Geometry: final body of the model. Coordinates: model frame, mm. Round coordinates to 2 decimals unless told otherwise and drop trailing zeros. Write each loop counter-clockwise with the first axis right and the second up, starting at its lowest first coordinate (ties: lowest second). Pieces come first, ordered by that corner, then holes. Notation, with made-up numbers: M 17.25,-38.75 L 46.25,-38.75 A27 cw 46.25,-22.75 Z; hole C 33.5,-5 d10. An arc over 180 degrees is marked long. Answer as CSV lines item,"result". Start each with the question number.
Q1. Section query C-C on z = 3.5. Output: boundary loops of the cut face in (x, y) (3 decimals).
Q2. First-contact query: pin 1 (1 mm diameter, centred on y = -2, z = 4.5, fed in from +X). Flat tip, straight axial feed; report the tip coordinate or a pass-through.
Q3. Section query B-B on y = 2.75. Output: boundary loops of the cut face in (x, z).
Q4. Section query A-A on x = 450.5. Output: boundary loops of the cut face in (y, z), and give its area (4 significant figures).
Q5. Ray query, probe 1 along Y at (x, z) = (378, 3.25); probe 2 along X at (y, z) = (0.75, 2.25); probe 3 along X at (y, z) = (3.5, 1). Return the intervals inside material, ascending.
```python
from build123d import *

# Parameters (mm, degrees)
RESSALTO_EXTRUS_O1_DEPTH = 6.25


with BuildPart() as part:
    # Esboço1 → Ressalto-extrusão1 (new body)
    with BuildSketch(Plane.XY.offset(6.25)):
        with BuildLine():
            Line((528.475, 6.5), (0, 6.5))
            ThreePointArc((0, 6.5), (-6.5, 0), (0, -6.5))
            Line((0, -6.5), (528.475, -6.5))
            ThreePointArc((528.475, -6.5), (534.975, 0), (528.475, 6.5))
        make_face()
        with BuildLine():
            Line((0, 4.848), (528.475, 4.848))
            ThreePointArc((528.475, 4.848), (533.323, 0), (528.475, -4.848))
            Line((528.475, -4.848), (0, -4.848))
            ThreePointArc((0, -4.848), (-4.848, 0), (0, 4.848))
        make_face(mode=Mode.SUBTRACT)
    extrude(amount=-RESSALTO_EXTRUS_O1_DEPTH)


solid = part.part
```
Entries:
1,outline,"M 0,-6.5 L 528.475,-6.5 A6.5 ccw 528.475,6.5 L 0,6.5 A6.5 ccw Z; hole M 0,-4.848 L 528.475,-4.848 A4.848 ccw 528.475,4.848 L 0,4.848 A4.848 ccw Z"
2,pin 1,"stops at x = 534.8"
3,outline,"M -5.89,0 L -3.99,0 L -3.99,6.25 L -5.89,6.25 Z; M 532.47,0 L 534.36,0 L 534.36,6.25 L 532.47,6.25 Z"
4,outline,"M -6.5,0 L -4.85,0 L -4.85,6.25 L -6.5,6.25 Z; M 4.85,0 L 6.5,0 L 6.5,6.25 L 4.85,6.25 Z"
4,area,"20.65 mm^2"
5,probe 1,"y = -6.5 to -4.85, 4.85 to 6.5"
5,probe 2,"x = -6.46 to -4.79, 533.26 to 534.93"
5,probe 3,"x = -5.48 to -3.35, 531.83 to 533.95"
